Here's how the part is built. I have some questions about the finished solid (model axes, mm). Face numbers are marked on the shaded views. Coordinates: 2 decimals unless noted, no trailing zeros. Answer as a JSON object with one key per item and string values. Group by question number.
1) If we mould it in two halves opening along X, with no side actions, what happens to the marked faces 1 and 2? For each: +X half, -X half, draft (parallel to the pull), parting line (faces both ways), or undercut.
2) I'm going to push flat-ended pins straight in: pin 1 (12 mm diameter, centred on x = 168.5, y = 57.5, fed in from +Z); pin 2 (4 mm diameter, centred on x = 522.5, z = -223, fed in from +Y); pin 3 (4 mm diameter, centred on x = 425, y = 157.5, fed in from -Z). Where does each tip first touch, or does it pass through?
3) I need wall thicknesses on probe 1 along Y at (x, z) = (32.5, -180.5); probe 2 along Z at (x, y) = (221.5, 175.5); probe 3 along X at (y, z) = (28, -187). Which ranges of each line are inside material? Lowest first, please. Write a range as [from, to].
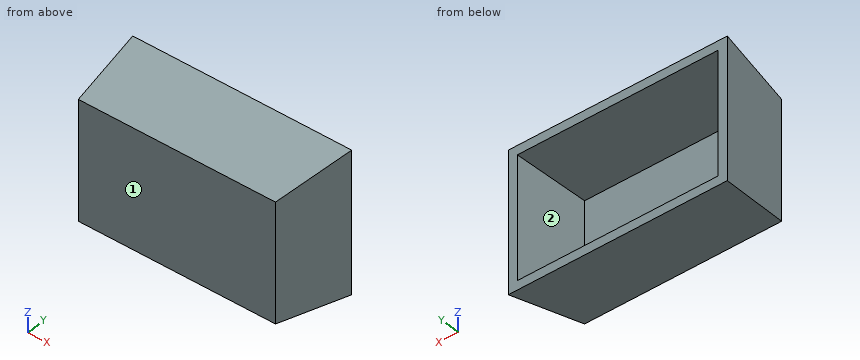
```python
from build123d import *

# Parameters (mm, degrees)
SHELL1_T           = -25.4
SKETCH5_W          = 929.67589299
SKETCH5_H          = 559.095756772
CUT_EXTRUDE1_DEPTH = 50.8


with BuildPart() as part:
    # Sketch2 → Loft1 section 0
    with BuildSketch(Plane(origin=(0, 266.7, 0), x_dir=(1, 0, 0), z_dir=(0, 1, 0))):
        with BuildLine():
            Line((-38.1, -38.1), (596.9, -38.1))
            Line((596.9, -38.1), (596.9, 368.3))
            Line((596.9, 368.3), (-38.1, 368.3))
            Line((-38.1, 368.3), (-38.1, -38.1))
        make_face()
    # Sketch1 → Loft1 section 1
    with BuildSketch(Plane(origin=(0, 0, 0), x_dir=(1, 0, 0), z_dir=(0, 1, 0))):
        with BuildLine():
            Line((0, 0), (558.8, 0))
            Line((558.8, 0), (558.8, 330.2))
            Line((558.8, 330.2), (0, 330.2))
            Line((0, 330.2), (0, 0))
        make_face()
    loft()

    # Shell1
    shell1_openings = [part.faces().sort_by_distance(p)[0] for p in [
        (279.4, 266.7, -165.1),
    ]]
    offset(amount=SHELL1_T, openings=shell1_openings, kind=Kind.INTERSECTION)

    # Sketch5 → Cut-Extrude1 (cut)
    with BuildSketch(Plane(origin=(0, 215.9, 0), x_dir=(1, 0, 0), z_dir=(0, 1, 0))):
        with Locations((273.30728983, 168.325552443)):
            Rectangle(SKETCH5_W, SKETCH5_H)
    extrude(amount=CUT_EXTRUDE1_DEPTH, mode=Mode.SUBTRACT)


solid = part.part
```
Determined:
{
 "1": {"face 1": "draft", "face 2": "undercut"},
 "2": {"pin 1": "z = 9.07", "pin 2": "y = 25.4", "pin 3": "z = -352.99"},
 "3": {"probe 1": "[0, 25.4]", "probe 2": "[-355.27, -329.61], [-0.59, 25.07]", "probe 3": "[-4, 21.66], [537.14, 562.8]"}
}
